Can you work these out from the drawing? Everything is in mm from the part's minimum corner. Round coordinates to 2 decimals unless told otherwise and drop trailing zeros. Write each loop counter-clockwise with the first axis right and the second up, starting at its lowest first coordinate (ties: lowest second). Pieces come first, ordered by that corner, then holes. Notation, with made-up numbers: (31, 74) - (58, 74) arc R28 cw to (58, 109) - close; hole circle Ø5 at (10.5, 8.5). An arc over 180 degrees is marked (long way). One line per item, written item: value. Start each with the question number.
Item 1: If I drill on line 1 (Y direction, x = 47, z = 2); line 2 (Z direction, x = 24, y = 162.5), over which ranges is the centre line in solid material (lowest first)?
Item 2: Imagine slicing it at B-B, the plane z = 42. Please give me the cut outline in (x, y), then the cut area to 3 significant figures.
Item 3: Imagine slicing it at A-A, the plane x = 6. Please give me the cut outline in (y, z).
Item 4: For P1, Ø2.5, axis at x = 26.5, y = 168, coming from the +Z side; P2, Ø1, axis at x = 24, z = 10.5, coming from the +Y side; P3, Ø3.5, axis at y = 164, z = 1.5, coming from the -X side, each with a flat end and sliding along its axis, tell me the tip position at first contact or that it passes through.
Item 5: Imagine slicing it at C-C, the plane z = 27. Please give me the cut outline in (x, y), then the cut area to 3 significant figures.
Item 6: Imagine slicing it at D-D, the plane x = 30.5. Please give me the cut outline in (y, z).
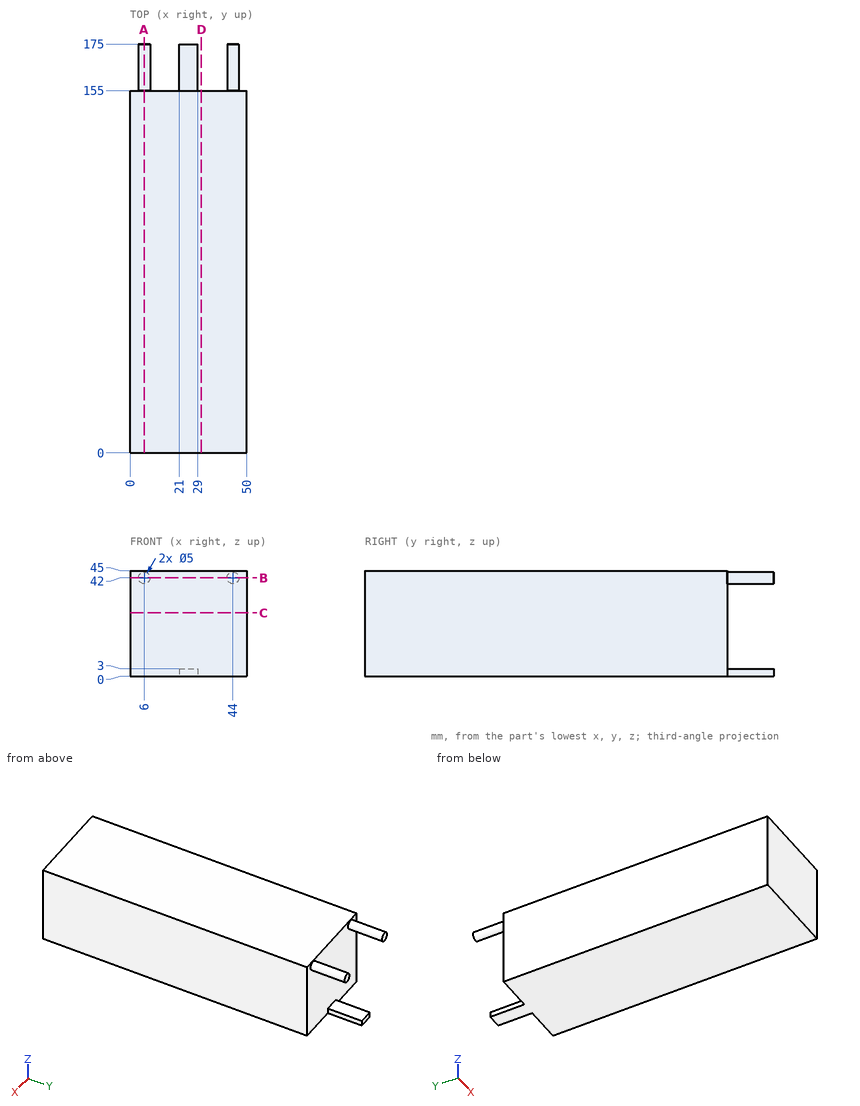
Values follow:
1. line 1: y = 0 to 155
1. line 2: z = 0 to 3
2. outline: (0, 0) - (50, 0) - (50, 155) - (46.5, 155) - (46.5, 175) - (41.5, 175) - (41.5, 155) - (8.5, 155) - (8.5, 175) - (3.5, 175) - (3.5, 155) - (0, 155) - close
2. area: 7,950 mm^2
3. outline: (0, 0) - (155, 0) - (155, 39.5) - (175, 39.5) - (175, 44.5) - (155, 44.5) - (155, 45) - (0, 45) - close
4. P1: stops at z = 3
4. P2: stops at y = 155
4. P3: stops at x = 21
5. outline: (0, 0) - (50, 0) - (50, 155) - (0, 155) - close
5. area: 7,750 mm^2
6. outline: (0, 0) - (155, 0) - (155, 45) - (0, 45) - close
